Here's how the part is built. I have some questions about the finished solid (model axes, mm). Face numbers are marked on the shaded views. A direction names the side the tool comes from. Coordinates: 2 decimals unless noted, no trailing zeros. Write each loop counter-clockwise with the first axis right and the second up, starting at its lowest first coordinate (ties: lowest second). Pieces come first, ordered by that corner, then holes. Notation, with made-up numbers: (-10, 23.5) -> (49, 23.5) arc R25 cw to (49, 37.5) -> close; hole circle Ø11 at (15.25, 58.25). An arc over 180 degrees is marked (long way). Put each result on its own line as item: value. Start each with the question number.
Item 1: For pin 1 (9.5 mm diameter, centred on x = 86, y = 17, fed in from +Z); pin 2 (10 mm diameter, centred on y = 5, z = 11, fed in from -X); pin 3 (3 mm diameter, centred on y = 16, z = 4, fed in from -X); pin 4 (1.2 mm diameter, centred on x = 5.5, z = 4, fed in from +Y), each with a flat end and sliding along its axis, tell me the tip position at first contact or that it passes through.
Item 2: If we mould it in two halves opening along X, with no side actions, what happens to the marked faces 6 and 7? For each: released by +X, released by -X, zero draft, split by the parting line, or undercut.
Item 3: On a 3-axis mill with a long thin cutter (end or side, diameter ignored), from which of +Z, -Z, +X, -X, +Y, -Y can I reach the whole of each face in a straight line? I mean the marked faces 1, 2, 3, 4 and 5. Say none if no direction works.
Item 4: I need wall thicknesses on line 1 (X direction, y = 3.5, z = 7); line 2 (X direction, y = 18, z = 3); line 3 (Y direction, x = 50, z = 16.25). Which ranges of each line are inside material? Lowest first, please. Write a range as [from, to].
Item 5: I want a section at C-C, the plane x = 9.5. List the corners of the cut face in (y, z) for me.
Item 6: I want a section at A-A, the plane z = 12.5. List the corners of the cut face in (x, y) for me.
Item 7: I want a section at B-B, the plane x = 45. List the corners of the cut face in (y, z) for me, then the cut area to 3 significant figures.
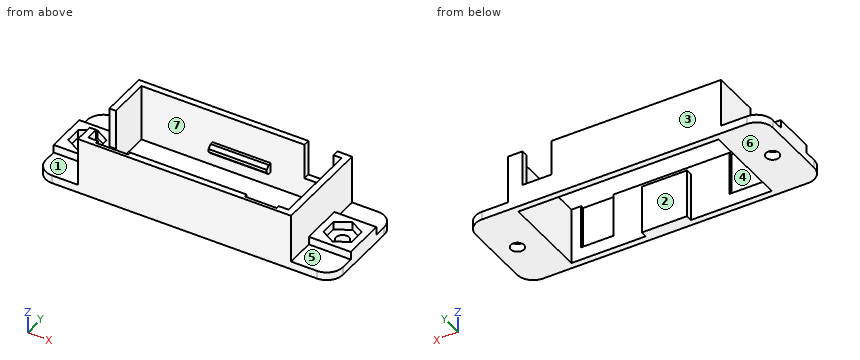
from build123d import *

# Parameters (mm, degrees)
F0_W      = 92
F0_H      = 31
F1_DEPTH  = 2.5
F2_W      = 66
F2_H      = 31
F2_W_2    = 62
F2_H_2    = 27
F3_DEPTH  = 15
F3_FACE_W = 62
F3_FACE_H = 27
F4_DEPTH  = 25
F5_W      = 13
F5_H      = 13
F6_DEPTH  = 2.5
F7_R      = 2.032
F8_DEPTH  = 5.001
F10_DEPTH = 2.5
F11_W     = 14
F11_H     = 2
F12_DEPTH = 15
F14_DEPTH = 2
F15_W     = 18
F15_H     = 3
F16_DEPTH = 2
F17_SIZE  = 1
F18_R     = 5
F19_W     = 10
F19_H     = 13.5
F20_DEPTH = 1
F21_W     = 9
F21_H     = 11
F22_DEPTH = 2


with BuildPart() as f1:
    # F0 (on Top) → F1 (new body)
    with BuildSketch(Plane.XY):
        with Locations((46, 15.5)):
            Rectangle(F0_W, F0_H)
    extrude(amount=F1_DEPTH)

    # F2 (on face) → F3 (join)
    with BuildSketch(Plane.XY.offset(2.5)):
        with Locations((46, 15.5)):
            Rectangle(F2_W, F2_H)
        with Locations((46, 15.5)):
            Rectangle(F2_W_2, F2_H_2, mode=Mode.SUBTRACT)
    extrude(amount=F3_DEPTH)

    # F3_face (on face) → F4 (cut)
    with BuildSketch(Plane(origin=(46, 15.5, 2.5), x_dir=(1, 0, 0), z_dir=(0, 0, 1))):
        Rectangle(F3_FACE_W, F3_FACE_H)
    extrude(amount=-F4_DEPTH, mode=Mode.SUBTRACT)

    # F5 (on face) → F6 (join)
    with BuildSketch(Plane.XY.offset(2.5)):
        with Locations((85.5, 15.5)):
            Rectangle(F5_W, F5_H)
        with Locations((6.5, 15.5)):
            Rectangle(F5_W, F5_H)
    extrude(amount=F6_DEPTH)

    # F7 (on face) → F8 (cut, through all)
    with BuildSketch(Plane.XY.offset(5)):
        with Locations((85.5, 15.5)):
            Circle(F7_R)
        with Locations((6.5, 15.5)):
            Circle(F7_R)
    extrude(amount=-F8_DEPTH, mode=Mode.SUBTRACT)

    # F9 (on face) → F10 (cut, through all)
    with BuildSketch(Plane.XY.offset(5)):
        Polygon((2.1, 18.040341), (2.1, 12.959659), (6.5, 10.419318), (10.9, 12.959659), (10.9, 18.040341), (6.5, 20.580682), align=None)
        Polygon((81.1, 12.959659), (85.5, 10.419318), (89.9, 12.959659), (89.9, 18.040341), (85.5, 20.580682), (81.1, 18.040341), align=None)
    extrude(amount=-F10_DEPTH, mode=Mode.SUBTRACT)

    # F11 (on Top) → F12 (join)
    with BuildSketch(Plane.XY):
        with Locations((47, 3)):
            Rectangle(F11_W, F11_H)
    extrude(amount=F12_DEPTH)

    # F13 (on face) → F14 (cut, through all)
    with BuildSketch(Plane(origin=(13, 0, 0), x_dir=(0, -1, 0), z_dir=(-1, 0, 0))):
        Polygon((-16, 17.5), (-16, 5), (-9, 5), (-6, 5), (-6, 17.5), align=None)
    extrude(amount=-F14_DEPTH, mode=Mode.SUBTRACT)

    # F15 (on face) → F16 (join)
    with BuildSketch(Plane.XZ.offset(-29)):
        with Locations((46, 6)):
            Rectangle(F15_W, F15_H)
    extrude(amount=F16_DEPTH)

    # F17
    f17_edges = [f1.edges().sort_by_distance(p)[0] for p in [
        (46, 27, 7.5),
        (46, 27, 4.5),
    ]]
    chamfer(f17_edges, length=F17_SIZE)

    # F18
    f18_edges = [f1.edges().sort_by_distance(p)[0] for p in [
        (0, 0, 1.25),
        (0, 31, 1.25),
        (92, 0, 1.25),
        (92, 31, 1.25),
    ]]
    fillet(f18_edges, radius=F18_R)

    # F19 (on face) → F20 (cut)
    with BuildSketch(Plane(origin=(0, 2, 0), x_dir=(-1, 0, 0), z_dir=(0, 1, 0))):
        with Locations((-69, 10.75)):
            Rectangle(F19_W, F19_H)
        with Locations((-23, 10.75)):
            Rectangle(F19_W, F19_H)
    extrude(amount=-F20_DEPTH, mode=Mode.SUBTRACT)

    # F21 (on face) → F22 (cut, through all)
    with BuildSketch(Plane(origin=(0, 31, 0), x_dir=(-1, 0, 0), z_dir=(0, 1, 0))):
        with Locations((-70, 12)):
            Rectangle(F21_W, F21_H)
    extrude(amount=-F22_DEPTH, mode=Mode.SUBTRACT)


solid = f1.part
Calculated:
1. pin 1: stops at z = 5
1. pin 2: stops at x = 13
1. pin 3: stops at x = 0
1. pin 4: stops at y = 22
2. face 6: zero draft
2. face 7: undercut
3. face 1: +Z, -X, -Y
3. face 2: +Z, -Z
3. face 3: +Z, -Z, +X, -X, +Y
3. face 4: +Z
3. face 5: +Z, +X, -Y
4. line 1: x = [13, 15], [40, 54], [77, 79]
4. line 2: x = [0, 2.1], [10.9, 15], [77, 81.1], [89.9, 92]
4. line 3: y = [0, 2], [29, 31]
5. outline: (0, 0) -> (31, 0) -> (31, 2.5) -> (22, 2.5) -> (22, 5) -> (18.85, 5) -> (18.85, 2.5) -> (12.15, 2.5) -> (12.15, 5) -> (9, 5) -> (9, 2.5) -> (0, 2.5) -> close
6. outline: (13, 0) -> (79, 0) -> (79, 31) -> (74.5, 31) -> (74.5, 29) -> (77, 29) -> (77, 2) -> (74, 2) -> (74, 1) -> (64, 1) -> (64, 2) -> (54, 2) -> (54, 4) -> (40, 4) -> (40, 2) -> (28, 2) -> (28, 1) -> (18, 1) -> (18, 2) -> (15, 2) -> (15, 6) -> (13, 6) -> close; (13, 16) -> (15, 16) -> (15, 29) -> (65.5, 29) -> (65.5, 31) -> (13, 31) -> close
7. outline: (0, 0) -> (4, 0) -> (4, 15) -> (2, 15) -> (2, 17.5) -> (0, 17.5) -> close; (27, 5.5) -> (28, 4.5) -> (29, 4.5) -> (29, 0) -> (31, 0) -> (31, 17.5) -> (29, 17.5) -> (29, 7.5) -> (28, 7.5) -> (27, 6.5) -> close
7. area: 105 mm2
